from build123d import *

# Parameters (mm, degrees)
SKETCH_1_W          = 10
SKETCH_1_H          = 10
EXTRUDE_1_DEPTH     = 10
SKETCH_2_R          = 1.5
CUT_EXTRUDE_1_DEPTH = 10
SKETCH_3_R          = 1.6
CUT_EXTRUDE_2_DEPTH = 10
SKETCH_4_R          = 1.6
CUT_EXTRUDE_3_DEPTH = 10


with BuildPart() as part:
    # 草图1 → 凸台-拉伸1 (new body)
    with BuildSketch(Plane(origin=(0, 0, 0), x_dir=(1, 0, 0), z_dir=(0, 1, 0))):
        with Locations((5, -5)):
            Rectangle(SKETCH_1_W, SKETCH_1_H)
    extrude(amount=EXTRUDE_1_DEPTH)

    # 草图2 → 切除-拉伸1 (cut)
    with BuildSketch(Plane.XY.offset(10)):
        with Locations((5, 5)):
            Circle(SKETCH_2_R)
    extrude(amount=-CUT_EXTRUDE_1_DEPTH, mode=Mode.SUBTRACT)

    # 草图3 → 切除-拉伸2 (cut)
    with BuildSketch(Plane(origin=(0, 10, 0), x_dir=(1, 0, 0), z_dir=(0, 1, 0))):
        with Locations(Location((5, -5, 0), (0, 0, 270))):
            Circle(SKETCH_3_R)
    extrude(amount=-CUT_EXTRUDE_2_DEPTH, mode=Mode.SUBTRACT)

    # 草图4 → 切除-拉伸3 (cut)
    with BuildSketch(Plane(origin=(10, 0, 0), x_dir=(0, 0, -1), z_dir=(1, 0, 0))):
        with Locations((-5, 5)):
            Circle(SKETCH_4_R)
    extrude(amount=-CUT_EXTRUDE_3_DEPTH, mode=Mode.SUBTRACT)


solid = part.part
Design review of the part built by this model. Coordinates are the model's own, in mm. Round coordinates to 2 decimals unless told otherwise and drop trailing zeros. Loops run counter-clockwise (first coordinate to the right, second up) from the corner with the lowest first, then second, coordinate; pieces in that order, holes last. Notation, with made-up numbers: M 29,8 L 37,8 A13 cw 37,12 Z; hole C -18,-22.75 d5. An arc over 180 degrees is marked long. Answer as a JSON object with one key per item and string values.
Item 1: We need section A-A on x = 5. Give the boundary of the cut face in (y, z), and give its area (3 significant figures).
Answer sheet:
{"outline": "M 0,0 L 3.5,0 L 3.5,3.4 L 0,3.4 Z; M 0,6.6 L 3.5,6.6 L 3.5,10 L 0,10 Z; M 6.5,0 L 10,0 L 10,3.4 L 6.5,3.4 Z; M 6.5,6.6 L 10,6.6 L 10,10 L 6.5,10 Z", "area": "47.6 mm^2"}
Item 2: Wall thickness on L1, parallel to Z at x = 7.6, y = 5; L2, parallel to X at y = 5, z = 2.55: over which ranges is each line inside the solid? List them lowest first. Write a range as from..to.
Answer sheet:
{"L1": "z = 0..3.4, 6.6..10", "L2": "x = 0..3.5, 6.5..10"}
Item 3: Clearance check with flat-ended pins moving along their axes: P1, Ø1.5, axis at x = 3, z = 4, coming from the -Y side; P2, Ø1.9, axis at x = 5, z = 5, coming from the -Y side. State where each tip first meets the part, or that it passes through.
Answer sheet:
{"P1": "stops at y = 0", "P2": "passes through"}
Item 4: The part is to be moulded in two halves that separate along X. For faces 1 (the flat face through (5, 10, 3)), 2 (the flat face through (10, 3, 5)), 3 (the cylindrical face through (5.07, 2, 3.4)), say which applies: pulls with the +X half, pulls with the -X half, needs draft (parallel to the pull), parting line crosses it, or undercut.
Answer sheet:
{"face 1": "needs draft", "face 2": "pulls with the +X half", "face 3": "undercut"}
Item 5: We need section C-C on z = 8. Give the boundary of the cut face in (x, y).
Answer sheet:
{"outline": "M 0,0 L 10,0 L 10,10 L 0,10 Z; hole C 5,5 d3"}
Item 6: We need section D-D on y = 3.25. Give the boundary of the cut face in (x, z), and give its area (3 significant figures).
Answer sheet:
{"outline": "M 0,0 L 10,0 L 10,10 L 0,10 Z; hole C 5,5 d3.2", "area": "92.0 mm^2"}
